Source: three-view drawing plus pictorial views. Frame: mm from the lowest corner of the part. A direction names the side the tool comes from. Round coordinates to 2 decimals unless told otherwise and drop trailing zeros. Loops run counter-clockwise (first coordinate to the right, second up) from the corner with the lowest first, then second, coordinate; pieces in that order, holes last. Notation, with made-up numbers: (-28, 89.25) -> (9, 89.25) arc R21 ccw to (9, 121.25) -> close; hole circle Ø2 at (11.5, 71.5). An arc over 180 degrees is marked (long way). Answer as a JSON object with one key per item and string values. Group by question number.
Item 1: Draft query along X for the marked faces 1, 2 and 3. Return one class per face: released by +X, released by -X, zero draft, split by the parting line, or undercut.
Item 2: Set-up query: the marked faces 4 and 5. Return all of +Z, -Z, +X, -X, +Y, -Y with unobstructed straight access to the full face (end or side cutting, diameter ignored); none if empty.
Item 3: Section query C-C on y = 38. Return loops of the section in (x, z), and give its area (3 significant figures).
Item 4: Section query B-B on z = 6. Return loops of the section in (x, y).
Item 5: Section query D-D on y = 53. Return loops of the section in (x, z), and give its area (3 significant figures).
Item 6: Material intervals for line 1 (X direction, y = 48, z = 2.5); line 2 (X direction, y = 19, z = 2.25); line 3 (Y direction, x = 55.5, z = 9.5) (3 decimals), sorted ascending. Write a range as [from, to].
Item 7: Pin query (flat end, axial travel): pin 1 (3 mm diameter, centred on y = 53, z = 3.5, fed in from +X). Return the tip coordinate at first contact, or that it passes through.
Item 8: Section query A-A on y = 18. Return loops of the section in (x, z).
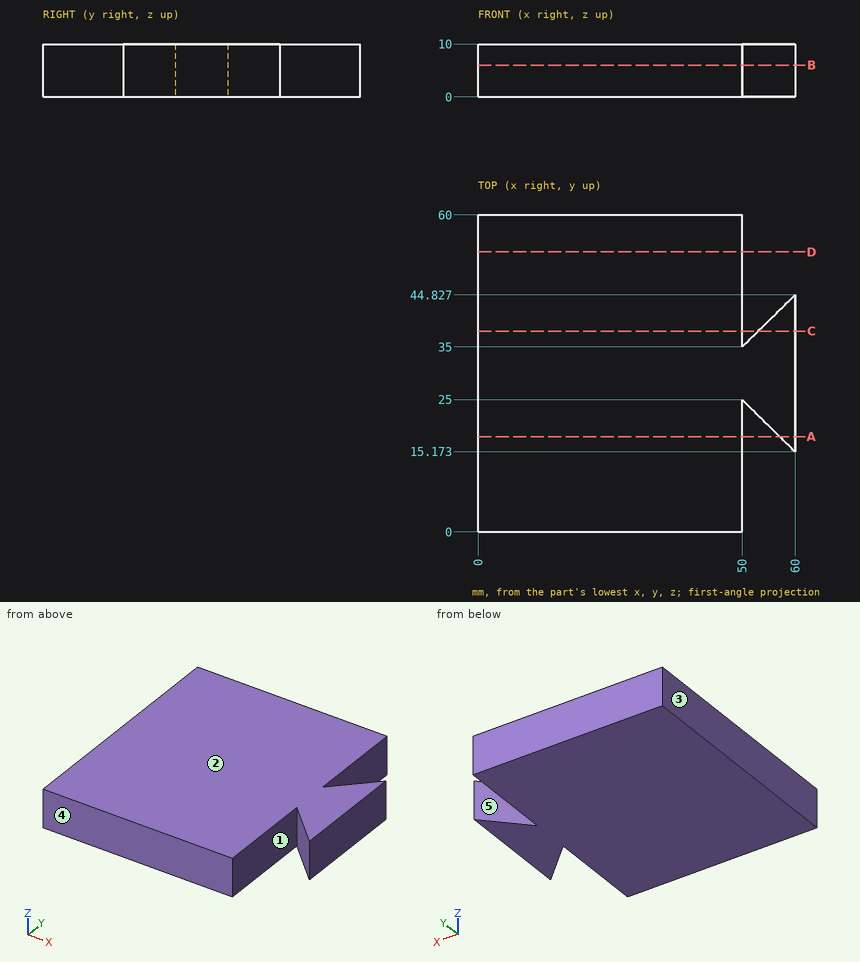
Solved:
{
 "1": {"face 1": "undercut", "face 2": "zero draft", "face 3": "released by -X"},
 "2": {"face 4": "+Z, -Z, +X, -X, -Y", "face 5": "+Z, -Z, +Y"},
 "3": {"outline": "(0, 0) -> (50, 0) -> (50, 10) -> (0, 10) -> close; (53.05, 0) -> (60, 0) -> (60, 10) -> (53.05, 10) -> close", "area": "569 mm²"},
 "4": {"outline": "(0, 0) -> (50, 0) -> (50, 25) -> (60, 15.17) -> (60, 44.83) -> (50, 35) -> (50, 60) -> (0, 60) -> close"},
 "5": {"outline": "(0, 0) -> (50, 0) -> (50, 10) -> (0, 10) -> close", "area": "500 mm²"},
 "6": {"line 1": "[0, 50]", "line 2": "[0, 50], [56.11, 60]", "line 3": "[19.595, 40.405]"},
 "7": {"pin 1": "x = 50"},
 "8": {"outline": "(0, 0) -> (50, 0) -> (50, 10) -> (0, 10) -> close; (57.12, 0) -> (60, 0) -> (60, 10) -> (57.12, 10) -> close"}
}
